Verification items for the finished model (mm, model axes). A direction names the side the tool comes from. Coordinates: 2 decimals unless noted, no trailing zeros. Order: outer loops, then holes, each group sorted by start corner. A loop starts at its lowest first (then second) coordinate and runs counter-clockwise, first axis right, second up. Notation, with made-up numbers: M 84.5,41 L 99.5,41 A17 cw 99.5,73 Z; hole C 11.5,34.5 d10. An arc over 180 degrees is marked long. Return JSON: item names as keys, results as strings. Group by question number.
1. Section check D-D, the plane y = 39.5. Record the cut outline in (x, z), plus the area to 3 significant figures.
2. Mould release check, pull along Z, two halves, no side actions. Record for faces 4 (the cylindrical face through (-19.076, 50.07, 6.007)), 5 (the cylindrical face through (7.66, -4.44, -18.475)), 6 (the flat face through (18, 45, -10)): +Z half, -Z half, draft (parallel to the pull), parting line (faces both ways), or undercut.
3. Section check C-C, the plane x = 0. Record the cut outline in (y, z), plus the area to 3 significant figures.
4. Set-up check for faces 1 (the flat face through (18, -45, -10)), 2 (the cylindrical face through (2.343, 48.591, 17.847)), 3 (the flat face through (0, 35, 0)): record each of +Z, -Z, +X, -X, +Y, -Y from which the full face is reachable in a straight line by a thin tool's end or side.
5. Section check B-B, the plane y = 16. Record the cut outline in (x, z), plus the area to 3 significant figures.
6. Material ranges on line 1 along Z through (x, y) = (-0.5, -21.5); line 2 along Z through (x, y) = (0, 50.75), recorded low to high.
7. Gauge pin test, flat ends, axial feed: pin 1 (2 mm diameter, centred on y = 38, z = 16, fed in from +X); pin 2 (6 mm diameter, centred on x = 13.5, z = 5.5, fed in from -Y); pin 3 (2 mm diameter, centred on x = 6.5, y = 15.5, fed in from -Z); pin 4 (10 mm diameter, centred on x = -0.5, y = 41, fed in from +Z). Record the tip position at first contact, or that the pin passes through.
8. Section check A-A, the plane z = 0. Record the cut outline in (x, y), plus the area to 3 significant figures.
```python
from build123d import *

# Parameters (mm, degrees)
F0_W     = 90
F0_H     = 2
F2_R     = 20
F3_DEPTH = 10
F4_R     = 18
F5_DEPTH = 13


with BuildPart() as f1:
    # F0 (on Right) → F1 (revolve)
    with BuildSketch(Plane.YZ):
        with Locations((0, -21)):
            Rectangle(F0_W, F0_H)
    revolve(axis=Axis((0, 40.8125, 0), (0, 1, 0)))

    # F2 (on face) → F3 (join, symmetric)
    with BuildSketch(Plane(origin=(0, 45, 0), x_dir=(-1, 0, 0), z_dir=(0, 1, 0))):
        Circle(F2_R)
    extrude(amount=F3_DEPTH, both=True)

    # F4 (on face) → F5 (cut)
    with BuildSketch(Plane(origin=(0, 55, 0), x_dir=(-1, 0, 0), z_dir=(0, 1, 0))):
        Circle(F4_R)
    extrude(amount=-F5_DEPTH, mode=Mode.SUBTRACT)


solid = f1.part
```
Answers follow:
{
 "1": {"outline": "C 0,0 d44", "area": "1,520 mm^2"},
 "2": {"face 4": "parting line", "face 5": "undercut", "face 6": "draft"},
 "3": {"outline": "M -45,-22 L 45,-22 L 45,-20 L 55,-20 L 55,-18 L 42,-18 L 42,18 L 55,18 L 55,20 L 45,20 L 45,22 L -45,22 L -45,20 L 35,20 L 35,-20 L -45,-20 Z", "area": "692 mm^2"},
 "4": {"face 1": "+Z, -Z, +X, -X, -Y", "face 2": "+Y", "face 3": "-Y"},
 "5": {"outline": "C 0,0 d44; hole C 0,0 d40", "area": "264 mm^2"},
 "6": {"line 1": "-21.99 to -19.99, 19.99 to 21.99", "line 2": "-20 to -18, 18 to 20"},
 "7": {"pin 1": "x = 16.09", "pin 2": "y = 35", "pin 3": "z = -21.3", "pin 4": "z = 22"},
 "8": {"outline": "M -22,-45 L -20,-45 L -20,35 L 20,35 L 20,-45 L 22,-45 L 22,45 L 20,45 L 20,55 L 18,55 L 18,42 L -18,42 L -18,55 L -20,55 L -20,45 L -22,45 Z", "area": "692 mm^2"}
}
